Here's how the part is built. I have some questions about the finished solid (model axes, mm). A direction names the side the tool comes from. Round coordinates to 2 decimals unless told otherwise and drop trailing zeros. Loops run counter-clockwise (first coordinate to the right, second up) from the corner with the lowest first, then second, coordinate; pieces in that order, holes last. Notation, with made-up numbers: M 10.25,-14 L 68.25,-14 A12 cw 68.25,1 Z; hole C 12.5,19.5 d5. An arc over 180 degrees is marked long. Write item = value, one per line. Start each with the question number.
from build123d import *

# Parameters (mm, degrees)
F0_R      = 3.5
F1_DEPTH  = 10
F0_W      = 31.4
F0_H      = 24
F2_DEPTH  = 15.7
F3_DEPTH  = 30.5
F6_DEPTH  = 100
F7_R      = 1.7
F7_R_2    = 5.2
F8_DEPTH  = 60
F9_DEPTH  = 100
F10_DEPTH = 100
F11_DEPTH = 10
F12_R     = 5
F0_R_2    = 1.7
F13_DEPTH = 6
F14_DEPTH = 6
F15_R     = 3.5
F15_R_2   = 1.4
F16_DEPTH = 16


# Not quite as in the source:
# - a feature names something its author has since deleted; it is built from what else it names


with BuildPart() as f1:
    # F0 (on Top) → F1 (new body)
    with BuildSketch(Plane.XY):
        Polygon((59.3, 50), (0, 50), (-59.3, 50), (-59.3, 26), (-12.5, 26), (-12.5, 5), (12.5, 5), (12.5, 26), (59.3, 26), align=None)
        with Locations((-53.3, 38)):
            Circle(F0_R, mode=Mode.SUBTRACT)
        with Locations((53.3, 38)):
            Circle(F0_R, mode=Mode.SUBTRACT)
    extrude(amount=F1_DEPTH)

    # F0 (on Top) → F2 (join)
    with BuildSketch(Plane.XY):
        with Locations((-75, 38)):
            Rectangle(F0_W, F0_H)
        with Locations((75, 38)):
            Rectangle(F0_W, F0_H)
    extrude(amount=F2_DEPTH)



with BuildPart() as f1b:
    # F0 (on Top) → F1, piece 2 (new body)
    with BuildSketch(Plane.XY):
        Polygon((12.5, -5), (-12.5, -5), (-12.5, -26), (-59.3, -26), (-59.3, -50), (0, -50), (59.3, -50), (59.3, -26), (12.5, -26), align=None)
        with Locations((-53.3, -38)):
            Circle(F0_R, mode=Mode.SUBTRACT)
        with Locations((53.3, -38)):
            Circle(F0_R, mode=Mode.SUBTRACT)
    extrude(amount=F1_DEPTH)

    # F0 (on Top) → F2, piece 2 (join)
    with BuildSketch(Plane.XY):
        with Locations((-75, -38)):
            Rectangle(F0_W, F0_H)
        with Locations((75, -38)):
            Rectangle(F0_W, F0_H)
    extrude(amount=F2_DEPTH)


with BuildPart() as f1_1:
    add(f1.part)

    add(f1b.part)  # F3 merges F1b
    # F0 (on Top) → F3 (join)
    with BuildSketch(Plane.XY):
        Polygon((12.5, 5), (-12.5, 5), (-12.5, 0), (-12.5, -5), (12.5, -5), (12.5, 0), align=None)
    extrude(amount=F3_DEPTH)

    # F4: union 

    # F5 (on face) → F6 (cut)
    with BuildSketch(Plane.XZ.offset(50)):
        with BuildLine():
            Line((59.3, 15.7), (59.3, 10))
            Line((59.3, 10), (60.936808709, 10))
            ThreePointArc((60.936808709, 10), (62.6266035374, 10.3294327596), (64.0689074703, 11.2694816254))
            ThreePointArc((64.0689074703, 11.2694816254), (69.1025794418, 14.5502725321), (75, 15.7))
            Line((75, 15.7), (59.3, 15.7))
        make_face()
        with BuildLine():
            ThreePointArc((82.7, 0), (75, 7.7), (67.3, 0))
            Line((67.3, 0), (82.7, 0))
        make_face()
        with BuildLine():
            ThreePointArc((-75, 15.7), (-69.1025794418, 14.5502725321), (-64.0689074703, 11.2694816254))
            ThreePointArc((-64.0689074703, 11.2694816254), (-62.6266035374, 10.3294327596), (-60.936808709, 10))
            Line((-60.936808709, 10), (-59.3, 10))
            Line((-59.3, 10), (-59.3, 15.7))
            Line((-59.3, 15.7), (-75, 15.7))
        make_face()
        with BuildLine():
            ThreePointArc((-67.3, 0), (-75, 7.7), (-82.7, 0))
            Line((-82.7, 0), (-67.3, 0))
        make_face()
    extrude(amount=-F6_DEPTH, mode=Mode.SUBTRACT)

    # F7 (on face) → F8 (cut, symmetric)
    with BuildSketch(Plane.XZ.offset(5)):
        with BuildLine():
            Line((-12.5, 30.5), (-12.5, 18))
            ThreePointArc((-12.5, 18), (-8.8388347819, 26.8388347478), (-4.83e-08, 30.5))
            Line((-4.83e-08, 30.5), (-12.5, 30.5))
        make_face()
        with BuildLine():
            Line((12.5, 30.5), (-4.83e-08, 30.5))
            ThreePointArc((-4.83e-08, 30.5), (8.8388347478, 26.8388347819), (12.5, 18))
            Line((12.5, 18), (12.5, 30.5))
        make_face()
        with BuildLine():
            add(Edge.make_bspline(
                [(-11.8176156762, 13.9264315731), (-11.6747882381, 13.1368398711), (-11.3919431578, 11.6323543495), (-12.1435697242, 10.5264146596), (-12.5, 10)],
                knots=[0, 0, 0, 0, 0.5238869887, 1, 1, 1, 1], degree=3))
            ThreePointArc((-11.8176156762, 13.9264315731), (-12.3282236343, 15.9348360783), (-12.5, 18))
            Line((-12.5, 18), (-12.5, 10))
        make_face()
        with BuildLine():
            Line((12.5, 10), (12.5, 18))
            ThreePointArc((12.5, 18), (12.3282236343, 15.9348360783), (11.8176156762, 13.9264315731))
            add(Edge.make_bspline(
                [(11.8176156762, 13.9264315731), (11.6747882381, 13.1368398711), (11.3919431578, 11.6323543495), (12.1435697242, 10.5264146596), (12.5, 10)],
                knots=[0, 0, 0, 0, 0.5238869887, 1, 1, 1, 1], degree=3))
        make_face()
        with Locations((-8, 18)):
            Circle(F7_R)
        with Locations((0, 26)):
            Circle(F7_R)
        with Locations((8, 18)):
            Circle(F7_R)
        with BuildLine():
            ThreePointArc((1.7, 10), (0, 11.7), (-1.7, 10))
            Line((-1.7, 10), (1.7, 10))
        make_face()
        with BuildLine():
            Line((1.7, 10), (-1.7, 10))
            ThreePointArc((-1.7, 10), (0, 8.3), (1.7, 10))
        make_face()
        with Locations((0, 18)):
            Circle(F7_R_2)
    extrude(amount=F8_DEPTH, both=True, mode=Mode.SUBTRACT)

    # F7 (on face) → F9 (cut)
    with BuildSketch(Plane.XZ.offset(5)):
        with BuildLine():
            Line((-1.7, 10), (-9.6046863561, 10))
            ThreePointArc((-9.6046863561, 10), (0, 5.5), (9.6046863561, 10))
            Line((9.6046863561, 10), (1.7, 10))
            ThreePointArc((1.7, 10), (0, 8.3), (-1.7, 10))
        make_face()
    extrude(amount=F9_DEPTH, mode=Mode.SUBTRACT)

    # F7 (on face) → F10 (cut)
    with BuildSketch(Plane.XZ.offset(5)):
        with BuildLine():
            Line((-1.7, 10), (-9.6046863561, 10))
            ThreePointArc((-9.6046863561, 10), (0, 5.5), (9.6046863561, 10))
            Line((9.6046863561, 10), (1.7, 10))
            ThreePointArc((1.7, 10), (0, 8.3), (-1.7, 10))
        make_face()
    extrude(amount=-F10_DEPTH, mode=Mode.SUBTRACT)

    # F7 (on face) → F11 (join)
    with BuildSketch(Plane.XZ.offset(5)):
        with BuildLine():
            Line((-1.7, 10), (-9.6046863561, 10))
            ThreePointArc((-9.6046863561, 10), (0, 5.5), (9.6046863561, 10))
            Line((9.6046863561, 10), (1.7, 10))
            ThreePointArc((1.7, 10), (0, 8.3), (-1.7, 10))
        make_face()
    extrude(amount=-F11_DEPTH)

    # F12
    f12_edges = [f1_1.edges().sort_by_distance(p)[0] for p in [
        (-12.5, 26, 5),
        (12.5, 26, 5),
        (-12.5, -26, 5),
        (12.5, -26, 5),
    ]]
    fillet(f12_edges, radius=F12_R)

    # F0 (on Top) → F13 (join)
    with BuildSketch(Plane.XY):
        Polygon((-90.7, 26), (-90.7, 50), (-99.7, 50), (-102.7, 50), (-102.7, 26), (-99.7, 26), align=None)
        with Locations((-96.7, 38)):
            Circle(F0_R_2, mode=Mode.SUBTRACT)
        Polygon((-90.7, -50), (-90.7, -26), (-99.7, -26), (-102.7, -26), (-102.7, -50), (-99.7, -50), align=None)
        with Locations((-96.7, -38)):
            Circle(F0_R_2, mode=Mode.SUBTRACT)
        Polygon((99.7, -26), (90.7, -26), (90.7, -50), (99.7, -50), (102.7, -50), (102.7, -26), align=None)
        with Locations((96.7, -38)):
            Circle(F0_R_2, mode=Mode.SUBTRACT)
        Polygon((99.7, 50), (90.7, 50), (90.7, 26), (99.7, 26), (102.7, 26), (102.7, 50), align=None)
        with Locations((96.7, 38)):
            Circle(F0_R_2, mode=Mode.SUBTRACT)
    extrude(amount=F13_DEPTH)

    # F0 (on Top) → F14 (join)
    with BuildSketch(Plane.XY):
        with Locations((-53.3, 38)):
            Circle(F0_R)
        with Locations((-53.3, 38)):
            Circle(F0_R_2, mode=Mode.SUBTRACT)
        with Locations((53.3, 38)):
            Circle(F0_R)
        with Locations((53.3, 38)):
            Circle(F0_R_2, mode=Mode.SUBTRACT)
        with Locations((-53.3, -38)):
            Circle(F0_R)
        with Locations((-53.3, -38)):
            Circle(F0_R_2, mode=Mode.SUBTRACT)
        with Locations((53.3, -38)):
            Circle(F0_R)
        with Locations((53.3, -38)):
            Circle(F0_R_2, mode=Mode.SUBTRACT)
    extrude(amount=F14_DEPTH)

    # F15 (on face) → F16 (join)
    with BuildSketch(Plane.XY.offset(15.7)):
        with Locations((-82.85, 38)):
            Circle(F15_R)
        with Locations((-82.85, 38)):
            Circle(F15_R_2, mode=Mode.SUBTRACT)
        with Locations((82.85, 38)):
            Circle(F15_R)
        with Locations((82.85, 38)):
            Circle(F15_R_2, mode=Mode.SUBTRACT)
        with Locations((82.85, -38)):
            Circle(F15_R)
        with Locations((82.85, -38)):
            Circle(F15_R_2, mode=Mode.SUBTRACT)
        with Locations((-82.85, -38)):
            Circle(F15_R)
        with Locations((-82.85, -38)):
            Circle(F15_R_2, mode=Mode.SUBTRACT)
    extrude(amount=F16_DEPTH)


solid = f1_1.part
Item 1: Please list where these lines run through material, in increasing order: line 1 (Y direction, x = -53.3, z = 2.3); line 2 (Z direction, x = 0, y = 0); line 3 (Y direction, x = -78, z = 11). Write a range as [from, to].
Item 2: We'd pull the mould along X, two halves only. Please class faces 1 (the flat face through (-102.7, -38, 3)), 2 (the flat face through (102.7, 38, 3)), 3 (the flat face through (-54, 36, 6)): released by +X, released by -X, zero draft, split by the parting line, or undercut.
Item 3: I want a section at A-A, the plane x = -36. List the corners of the cut face in (y, z) for me, then the cut area to 3 significant figures.
Item 4: I want a section at D-D, the plane y = -19. List the corners of the cut face in (x, z) for me, then the cut area to 3 significant figures.
Item 5: For faces 4 (the cylindrical face through (-85.4, -35.6, 23.6)), 5 (the flat face through (-61, 26, 6)), 6 (the cylindrical face through (14, -24.57, 5.07)), which set-ups out of +Z, -Z, +X, -X, +Y, -Y let a thin tool reach every point of the face, with its end or its side?
Item 6: I want a section at B-B, the plane y = -29. List the corners of the cut face in (x, z) for me.
Item 7: Will these pins go through, and if not, where does the flat tip stop? pin 1 Ø3 at (y, z) = (16, 6) entering from -X; pin 2 Ø6 at (x, y) = (98, 36.5) entering from +Z; pin 3 Ø3 at (y, z) = (42, 9) entering from +X.
Item 8: I want a section at C-C, the plane x = -70. List the corners of the cut face in (y, z) for me.
Worked out:
q1.line_1 = [-50, -39.7], [-36.3, -26], [26, 36.3], [39.7, 50]
q1.line_2 = [0, 8.3], [11.7, 12.8], [23.2, 24.3], [27.7, 30.5]
q1.line_3 = [-50, -26], [26, 50]
q2.face_1 = released by -X
q2.face_2 = released by +X
q2.face_3 = undercut
q3.outline = M -50,0 L -26,0 L -26,10 L -50,10 Z; M 26,0 L 50,0 L 50,10 L 26,10 Z
q3.area = 480 mm2
q4.outline = M -12.5,0 L 12.5,0 L 12.5,10 L 9.6,10 A12.5 cw -9.6,10 L -12.5,10 Z
q4.area = 190 mm2
q5.face_4 = +Z
q5.face_5 = +Z, -Z, -X
q5.face_6 = +Z, -Z, +X
q6.outline = M -102.7,0 L -82.7,0 A7.7 cw -67.3,0 L 67.3,0 A7.7 cw 82.7,0 L 102.7,0 L 102.7,6 L 90.7,6 L 90.7,15.7 L 75,15.7 A15.7 ccw 64.07,11.27 A4.5 cw 60.94,10 L 9.6,10 A12.5 cw -9.6,10 L -60.94,10 A4.5 cw -64.07,11.27 A15.7 ccw -75,15.7 L -90.7,15.7 L -90.7,6 L -102.7,6 Z
q7.pin_1 = -12.5
q7.pin_2 = 6
q7.pin_3 = 90.7
q8.outline = M -50,5.86 L -26,5.86 L -26,14.88 L -50,14.88 Z; M 26,5.86 L 50,5.86 L 50,14.88 L 26,14.88 Z
